Autodesk Inventor part; units mm, degrees
ref_plane "YZ Plane" through (0, 0, 0) normal (1, 0, 0) x (0, 1, 0)
ref_plane "XZ Plane" through (0, 0, 0) normal (0, 1, 0) x (-1, 0, 0)
ref_plane "XY Plane" through (0, 0, 0) normal (0, 0, 1) x (1, 0, 0)
sketch "Szkic1" plane through (0, 0, 0) normal (0, 1, 0) x (-1, 0, 0)
  line L0 (0, 0) -> (10, 0)
  line L1 (10, 0) -> (10, -5.7)
  line L2 (10, -5.7) -> (0, -5.7)
  line L3 (0, -5.7) -> (0, 0)
  dimension "d0" = 10
  dimension "d1" = 5.7
extrude "Wyciągnięcie proste1" add sketch "Szkic1" along normal blind 2.6
sketch "Szkic2" plane through (-10, 0, 0) normal (0, 0, 1) x (1, 0, 0)
  line L0 (0, 0) -> (10, 0)
  line L1 (10, 0) -> (10, 2.6)
  line L2 (0, 2.6) -> (10, 2.6)
  line L3 (0, 0) -> (0, 2.6)
  line L4 (0, 0) -> (0, 2.6)
  line L5 (10, 0) -> (0, 0)
  line L6 (0, 2.6) -> (2.7, 2.6)
  line L7 (2.7, 2.6) -> (2.7, 0)
  line L8 (2.7, 0) -> (0, 0)
  line L9 (0, 0) -> (0, 2.6)
  line L10 (10, 2.6) -> (0, 2.6)
  line L11 (2.7, 0) -> (5, 0)
  line L12 (5, 0) -> (5, 2.6)
  line L13 (5, 2.6) -> (2.7, 2.6)
  line L14 (2.7, 2.6) -> (2.7, 0)
  dimension "d4" = 2.7
extrude "Wyciągnięcie proste2" add sketch "Szkic2" along normal blind 0.42 contours L7 L2 L12 L0
chamfer "Faza1" distance 0.4 angle 45 2 edges at (-6.15, 2.6, 0.42) (-6.15, 0, 0.42)
properties part number "wlacznik"
The listing builds one solid part. Answer for the finished solid, in the listing's coordinates (mm). A direction names the side the tool comes from. Coordinates: 2 decimals unless noted, no trailing zeros. Loops run counter-clockwise (first coordinate to the right, second up) from the corner with the lowest first, then second, coordinate; pieces in that order, holes last. Notation, with made-up numbers: (38.5, 79.5) -> (68.5, 79.5) arc R19 cw to (68.5, 97.5) -> close; hole circle Ø10 at (68, 55.5). An arc over 180 degrees is marked (long way). Answer in a Markdown table with one row per item. Add a question column.
1. Consider line 1 (Z direction, x = -2, y = 2.1). Determine where the line is inside the solid, lowest interval first. Write a range as [from, to].
2. For faces 1 (the flat face through (-5, 0, -3)), 2 (the flat face through (-9, 1, 0)), 3 (the flat face through (-2, 1, 0)), determine the directions among +Z, -Z, +X, -X, +Y, -Y from which every point of the face is accessible in a straight line to the end or side of a thin tool.
3. The part is cut by section B-B, the plane x = -9. Write down the section's boundary in (y, z), then the cut area to 3 significant figures.
4. The part is cut by section C-C, the plane y = 1.55. Write down the section's boundary in (x, z).
5. The part is cut by section A-A, the plane y = 2.3. Write down the section's boundary in (x, z).
Answer below:
| question | item | result |
|---|---|---|
| 1 | line 1 | [-5.7, 0] |
| 2 | face 1 | +Z, -Z, +X, -X, -Y |
| 2 | face 2 | +Z, -X, +Y, -Y |
| 2 | face 3 | +Z, +X, +Y, -Y |
| 3 | outline | (0, -5.7) -> (2.6, -5.7) -> (2.6, 0) -> (0, 0) -> close |
| 3 | area | 14.8 mm2 |
| 4 | outline | (-10, -5.7) -> (0, -5.7) -> (0, 0) -> (-5, 0) -> (-5, 0.42) -> (-7.3, 0.42) -> (-7.3, 0) -> (-10, 0) -> close |
| 5 | outline | (-10, -5.7) -> (0, -5.7) -> (0, 0) -> (-5, 0) -> (-5, 0.32) -> (-7.3, 0.32) -> (-7.3, 0) -> (-10, 0) -> close |
